from build123d import *

# Parameters (mm, degrees)
SKETCH1_W           = 615.95
SKETCH1_H           = 130.175
BOSS_EXTRUDE1_DEPTH = 3.175
SKETCH2_R           = 1.25
SKETCH2_R_2         = 12.7
SKETCH2_R_3         = 8
SKETCH2_W           = 73.66
SKETCH2_H           = 24.13
CUT_EXTRUDE1_DEPTH  = 315.793684667


with BuildPart() as part:
    # Sketch1 → Boss-Extrude1 (new body)
    with BuildSketch(Plane(origin=(0, 0, 0), x_dir=(1, 0, 0), z_dir=(0, 1, 0))):
        Rectangle(SKETCH1_W, SKETCH1_H)
    extrude(amount=BOSS_EXTRUDE1_DEPTH)

    # Sketch2 → Cut-Extrude1 (cut, through all)
    with BuildSketch(Plane(origin=(0, 3.175, 0), x_dir=(1, 0, 0), z_dir=(0, 1, 0))):
        with Locations(Location((41.099999842, 9.699999904, 0), (0, 0, 270))):
            Circle(SKETCH2_R)
        with Locations(Location((41.099999842, -22.399999904, 0), (0, 0, 90))):
            Circle(SKETCH2_R)
        with Locations(Location((-41.099999842, -22.399999904, 0), (0, 0, 270))):
            Circle(SKETCH2_R)
        with Locations(Location((-41.099999842, 9.699999904, 0), (0, 0, 90))):
            Circle(SKETCH2_R)
        with Locations(Location((-76.2, -6.35, 0), (0, 0, 270))):
            Circle(SKETCH2_R_2)
        with Locations(Location((-93.98, -6.35, 0), (0, 0, 270))):
            Circle(SKETCH2_R)
        with Locations(Location((-58.42, -6.35, 0), (0, 0, 270))):
            Circle(SKETCH2_R)
        with Locations(Location((86.2, 6.15, 0), (0, 0, 270))):
            Circle(SKETCH2_R)
        with Locations(Location((86.2, -18.85, 0), (0, 0, 270))):
            Circle(SKETCH2_R)
        with Locations(Location((66.2, -18.85, 0), (0, 0, 270))):
            Circle(SKETCH2_R)
        with Locations(Location((66.2, 6.15, 0), (0, 0, 270))):
            Circle(SKETCH2_R)
        with Locations(Location((76.2, -6.35, 0), (0, 0, 270))):
            Circle(SKETCH2_R_3)
        with Locations(Location((246.38, -6.35, 0), (0, 0, 90))):
            Circle(SKETCH2_R)
        with Locations(Location((210.82, -6.35, 0), (0, 0, 90))):
            Circle(SKETCH2_R)
        with Locations(Location((228.6, -6.35, 0), (0, 0, 90))):
            Circle(SKETCH2_R_2)
        with Locations((0, -6.35)):
            Rectangle(SKETCH2_W, SKETCH2_H)
    extrude(amount=-CUT_EXTRUDE1_DEPTH, mode=Mode.SUBTRACT)


solid = part.part
The model under review builds one solid part; all positions refer to its coordinate system, in mm. Round coordinates to 2 decimals unless told otherwise and drop trailing zeros. Write item = value, one per line. Start each with the question number.
Item 1: Take a section at A-A on y = 1.1. Count the separate pieces of the cut face and the enclosed holes in it, plus the area to 3 significant figures.
Item 2: Mouldability with a two-part tool opening along Z and no side actions: class faces 1 (the cylindrical face through (68.39, 1.61, 4.62)), 2 (the flat face through (-4, 0, -15)) as released by +Z, released by -Z, zero draft, split by the parting line, or undercut.
Item 3: To check wall thickness, follow L1, parallel to X at y = 1.85, z = -9.7 (3 decimals); L2, parallel to Z at x = -31, y = 2.6 (1 decimal); L3, parallel to Z at x = 237.5, y = 3. State the ranges of each line that lie inside material, in increasing order.
Result:
q1.separate_pieces = 1
q1.enclosed_holes = 16
q1.area = 77,100 mm²
q2.face_1 = undercut
q2.face_2 = zero draft
q3.L1 = -307.975 to -42.35, -39.85 to 39.85, 42.35 to 307.975
q3.L2 = -65.1 to -5.7, 18.4 to 65.1
q3.L3 = -65.09 to -2.71, 15.41 to 65.09
